The model under review builds one solid part; all positions refer to its coordinate system, in mm. A direction names the side the tool comes from. Coordinates: 2 decimals unless noted, no trailing zeros. Write each loop counter-clockwise with the first axis right and the second up, starting at its lowest first coordinate (ties: lowest second). Pieces come first, ordered by that corner, then holes. Notation, with made-up numbers: (-18.5, 64.25) - (37.5, 64.25) arc R25 ccw to (37.5, 98.25) - close; hole circle Ø3 at (55, 9). An arc over 180 degrees is marked (long way). Put each result on its own line as item: value. Start each with the question number.
Item 1: Machinability: for faces 5 (the face through (-26, 64.12, -47)), 6 (the face through (1, 153.12, 1)), which of the approach directions +Z, -Z, +X, -X, +Y, -Y give a long, thin tool a straight path to every point of the face, cutting with its end or side? Answer none if there is none.
Item 2: Mouldability with a two-part tool opening along Y and no side actions: class faces 1 (the face through (7.58, 99.05, -57.74)), 2 (the face through (11.54, 29.05, 51.97)), 3 (the face through (11.54, 69.05, 51.97)), 4 (the face through (1, 0, 1)) as pulls with the +Y half, pulls with the -Y half, needs draft (parallel to the pull), parting line crosses it, or undercut.
Item 3: Consider section B-B on y = 16. Give the boundary of the cut face in (x, z) (3 decimals), then the cut area to 3 significant figures.
Item 4: To check wall thickness, follow L1, parallel to X at y = 46, z = 1; L2, parallel to Z at x = -33.5, y = 10.5; L3, parallel to Z at x = -12.5, y = 15.5. State the ranges of each line that lie inside material, in increasing order. Write a range as [from, to].
Item 5: For pin 1 (2 mm diameter, centred on x = 7.5, y = 87, fed in from -Z); pin 2 (1 mm diameter, centred on y = 53, z = 36.5, fed in from -X); pin 3 (2 mm diameter, centred on y = 70.5, z = 12.5, fed in from -X); pin 4 (6 mm diameter, centred on x = 20.5, z = -13, fed in from -Y), all flat-tipped, find the tip position at first contact; note any pin that passes through.
Item 6: Consider section A-A on y = 67.5. Give the boundary of the cut face in (x, z) (3 decimals).
Autodesk Fusion 360 part; units mm, degrees
sketch "Sketch1" plane through (0, 0, 0) normal (0, 0, 1) x (1, 0, 0)
sketch "Sketch2" plane through (0, 0, 0) normal (0, 0, 1) x (1, 0, 0)
sketch "Sketch3" plane through (0, 0, 0) normal (0, 0, 1) x (1, 0, 0)
  line L0 (0, 0) -> (0, 153.12)
  line L1 (-58.235, 153.12) -> (-58.235, 114.12)
  line L2 (-58.235, 114.12) -> (-53.235, 114.12)
  line L3 (-53.235, 114.12) -> (-53.235, 104.12)
  line L4 (-53.235, 104.12) -> (-58.235, 104.12)
  line L5 (-58.235, 104.12) -> (-58.235, 94.12)
  line L6 (-58.235, 94.12) -> (-53.235, 94.12)
  line L7 (-53.235, 94.12) -> (-53.235, 84.12)
  line L8 (-53.235, 84.12) -> (-58.235, 84.12)
  line L9 (-58.235, 84.12) -> (-58.235, 74.12)
  line L10 (-58.235, 74.12) -> (-53.235, 74.12)
  line L11 (-53.235, 74.12) -> (-53.235, 64.12)
  line L12 (-53.235, 64.12) -> (-58.235, 64.12)
  line L13 (-58.235, 64.12) -> (-58.235, 54.12)
  line L14 (-58.235, 54.12) -> (-53.235, 54.12)
  line L15 (-53.235, 54.12) -> (-53.235, 44.12)
  line L16 (-53.235, 44.12) -> (-58.235, 44.12)
  line L17 (-58.235, 44.12) -> (-58.235, 34.12)
  line L18 (-58.235, 34.12) -> (-53.235, 34.12)
  line L19 (-53.235, 34.12) -> (-53.235, 24.12)
  line L20 (-53.235, 24.12) -> (-58.235, 24.12)
  line L21 (-58.235, 24.12) -> (-58.235, 5.0228)
  line L22 (-58.235, 5.0228) -> (-58.235, 0)
  line L23 (-58.235, 153.12) -> (0, 153.12)
  line L24 (-58.235, 0) -> (0, 0)
  dimension "d4" = 153.12
  dimension "d5" = 58.235
  dimension "d6" = 39
  dimension "d7" = 5
  dimension "d8" = 10
  dimension "d9" = 5
  dimension "d10" = 10
  dimension "d11" = 5
  dimension "d12" = 10
  dimension "d13" = 5
  dimension "d14" = 10
  dimension "d15" = 5
  dimension "d16" = 10
  dimension "d17" = 5
  dimension "d18" = 10
  dimension "d19" = 5
  dimension "d20" = 10
  dimension "d21" = 5
  dimension "d22" = 10
  dimension "d23" = 5
  dimension "d24" = 10
  dimension "d25" = 5
revolve "Revolve1" add sketch "Sketch3" angle 360 about axis through (0, 0, 0) along (0, 1, 0)
Report:
1. face 5: none
1. face 6: +Z, -Z, +X, -X, +Y
2. face 1: needs draft
2. face 2: undercut
2. face 3: undercut
2. face 4: pulls with the -Y half
3. outline: circle Ø116.47 at (0, 0)
3. area: 10,700 mm²
4. L1: [-53.23, 53.23]
4. L2: [-47.63, 47.63]
4. L3: [-56.88, 56.88]
5. pin 1: z = -52.84
5. pin 2: x = -39.22
5. pin 3: x = -51.98
5. pin 4: y = 0
6. outline: circle Ø106.47 at (0, 0)
